from build123d import *

# Parameters (mm, degrees)
SKETCH1_W           = 203.2
SKETCH1_H           = 127
BOSS_EXTRUDE1_DEPTH = 3.175
CUT_EXTRUDE1_DEPTH  = 3.175


with BuildPart() as part:
    # Sketch1 → Boss-Extrude1 (new body)
    with BuildSketch(Plane(origin=(0, 0, 0), x_dir=(1, 0, 0), z_dir=(0, 1, 0))):
        Rectangle(SKETCH1_W, SKETCH1_H)
    extrude(amount=BOSS_EXTRUDE1_DEPTH)

    # Sketch3 → Cut-Extrude1 (cut)
    with BuildSketch(Plane(origin=(0, 3.175, 0), x_dir=(1, 0, 0), z_dir=(0, 1, 0))):
        Polygon((-98.425, 12.7), (-101.6, 12.7), (-101.6, 63.5), (-20.32, 63.5), (-20.32, 60.325), (-98.425, 60.325), align=None)
        Polygon((20.32, 60.325), (98.425, 60.325), (98.425, 12.7), (101.6, 12.7), (101.6, 63.5), (20.32, 63.5), align=None)
        Polygon((-101.6, -12.7), (-101.6, -65.513366778), (-20.32, -63.5), (-20.32, -60.325), (-98.425, -60.325), (-98.425, -12.7), align=None)
        Polygon((20.32, -60.325), (20.32, -63.5), (101.6, -63.5), (101.6, -12.7), (98.425, -12.7), (98.425, -60.325), align=None)
    extrude(amount=-CUT_EXTRUDE1_DEPTH, mode=Mode.SUBTRACT)


solid = part.part
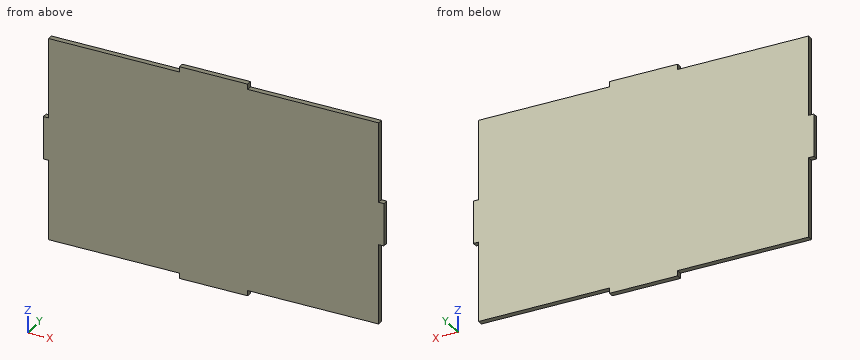
Part model, mm, in its own coordinate system. Give positions to 0.01 mm unless a question says otherwise; leave off trailing zeros. Loops run counter-clockwise (first coordinate to the right, second up) from the corner with the lowest first, then second, coordinate; pieces in that order, holes last.
(1) Band-saw the part on B-B (z = 28.5). Write the cut outline in (x, y) (3 decimals), and give its area (3 significant figures).
Return value:
outline: (-98.425, 0) - (98.425, 0) - (98.425, 3.175) - (-98.425, 3.175) - close
area: 625 mm2
(2) Band-saw the part on C-C (x = -36). Write the cut outline in (y, z) (3 decimals), and give its area (3 significant figures).
Return value:
outline: (0, -60.325) - (3.175, -60.325) - (3.175, 60.325) - (0, 60.325) - close
area: 383 mm2
(3) Drill centre lines: line 1 along Z through (x, y) = (73, 2.1) (3 decimals); line 2 along X through (y, z) = (2.4, 32) (3 decimals). Where is each one in solid material? Low to high.
Return value:
line 1: z = -60.325 to 60.325
line 2: x = -98.425 to 98.425
(4) Band-saw the part on A-A (y = 2.3). Write the cut outline in (x, z) (3 decimals), and give its area (3 significant figures).
Return value:
outline: (-101.6, -12.7) - (-98.425, -12.7) - (-98.425, -60.325) - (-20.32, -60.325) - (-20.32, -63.5) - (20.32, -63.5) - (20.32, -60.325) - (98.425, -60.325) - (98.425, -12.7) - (101.6, -12.7) - (101.6, 12.7) - (98.425, 12.7) - (98.425, 60.325) - (20.32, 60.325) - (20.32, 63.5) - (-20.32, 63.5) - (-20.32, 60.325) - (-98.425, 60.325) - (-98.425, 12.7) - (-101.6, 12.7) - close
area: 24,200 mm2
(5) Pin check, flat tips, straight feed: pin 1 (1 mm diameter, centred on y = 2, z = 46.5, fed in from -X) (3 decimals); pin 2 (1 mm diameter, centred on x = -99.5, y = 1, fed in from -Z); pin 3 (1.5 mm diameter, centred on y = 2.5, z = -35.5, fed in from +X) (3 decimals). Stop position of each tip, or through.
Return value:
pin 1: stops at x = -98.425
pin 2: stops at z = -12.7
pin 3: stops at x = 98.425
